Can you work these out from the model? Positions are in its coordinate system, mm. Face numbers are marked on the shaded views. A direction names the side the tool comes from. Give positions to 0.01 mm unless a question says otherwise; leave off trailing zeros. Order: outer loops, then holes, each group sorted by start corner. A loop starts at its lowest first (then second) coordinate and runs counter-clockwise, first axis right, second up. Notation, with made-up numbers: (-16.5, 55) -> (18.5, 55) arc R6 ccw to (18.5, 62) -> close; hole circle Ø8 at (19, 23). An arc over 180 degrees is marked (long way). Answer as CSV lines item,"result".
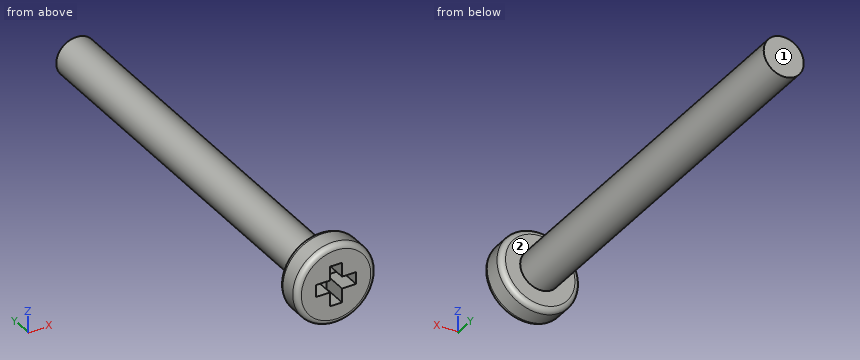
```python
from build123d import *

# Parameters (mm, degrees)
SKETCH1_R           = 3
BOSS_EXTRUDE1_DEPTH = 2
SKETCH2_R           = 1.5
BOSS_EXTRUDE2_DEPTH = 30
SKETCH3_W           = 0.9
SKETCH3_H           = 0.9
SKETCH3_W_2         = 1.05
SKETCH3_H_2         = 1.05
CUT_EXTRUDE1_DEPTH  = 1.9
FILLET1_R           = 0.4


with BuildPart() as part:
    # Sketch1 → Boss-Extrude1 (new body)
    with BuildSketch(Plane(origin=(0, 0, 0), x_dir=(1, 0, 0), z_dir=(0, 1, 0))):
        Circle(SKETCH1_R)
    extrude(amount=BOSS_EXTRUDE1_DEPTH)

    # Sketch2 → Boss-Extrude2 (add)
    with BuildSketch(Plane(origin=(0, 2, 0), x_dir=(1, 0, 0), z_dir=(0, 1, 0))):
        Circle(SKETCH2_R)
    extrude(amount=BOSS_EXTRUDE2_DEPTH)

    # Sketch3 → Cut-Extrude1 (cut)
    with BuildSketch(Plane(origin=(0, 0, 0), x_dir=(-1, 0, 0), z_dir=(0, -1, 0))):
        Rectangle(SKETCH3_W, SKETCH3_H)
        with Locations((0.975, 0)):
            Rectangle(SKETCH3_W_2, SKETCH3_H)
        with Locations((0, -0.975)):
            Rectangle(SKETCH3_W, SKETCH3_H_2)
        with Locations((-0.975, 0)):
            Rectangle(SKETCH3_W_2, SKETCH3_H)
        with Locations((0, 0.975)):
            Rectangle(SKETCH3_W, SKETCH3_H_2)
    extrude(amount=-CUT_EXTRUDE1_DEPTH, mode=Mode.SUBTRACT)

    # Fillet1
    fillet1_edges = [part.edges().sort_by_distance(p)[0] for p in [
        (-3, 0, 0),
        (-3, 2, 0),
    ]]
    fillet(fillet1_edges, radius=FILLET1_R)


solid = part.part
```
Item 1: Imagine slicing it at A-A, the plane z = 0. Please give me the cut outline in (x, y), then the cut area to 3 significant figures.
Numbers:
outline,"(-3, 0.4) arc R0.4 ccw to (-2.6, 0) -> (-1.5, 0) -> (-1.5, 1.9) -> (1.5, 1.9) -> (1.5, 0) -> (2.6, 0) arc R0.4 ccw to (3, 0.4) -> (3, 1.6) arc R0.4 ccw to (2.6, 2) -> (1.5, 2) -> (1.5, 32) -> (-1.5, 32) -> (-1.5, 2) -> (-2.6, 2) arc R0.4 ccw to (-3, 1.6) -> close"
area,"96.2 mm²"
Item 2: Imagine slicing it at C-C, the plane y = 26. Please give me the cut outline in (x, z), then the cut area to 3 significant figures.
Numbers:
outline,"circle Ø3 at (0, 0)"
area,"7.07 mm²"
Item 3: For the marked faces 1 and 2, which set-ups out of +Z, -Z, +X, -X, +Y, -Y let a thin tool reach every point of the face, with its end or its side?
Numbers:
face 1,"+Z, -Z, +X, -X, +Y"
face 2,"+Y"
Item 4: Imagine slicing it at B-B, the plane x = 0. Please give me the cut outline in (y, z).
Numbers:
outline,"(0, -2.6) arc R0.4 ccw to (0.4, -3) -> (1.6, -3) arc R0.4 ccw to (2, -2.6) -> (2, -1.5) -> (32, -1.5) -> (32, 1.5) -> (2, 1.5) -> (2, 2.6) arc R0.4 ccw to (1.6, 3) -> (0.4, 3) arc R0.4 ccw to (0, 2.6) -> (0, 1.5) -> (1.9, 1.5) -> (1.9, -1.5) -> (0, -1.5) -> close"
Item 5: Please list where these lines run through material, in increasing order: line 1 along Y through (x, z) = (1.15, -2.2); line 2 along Y through (x, z) = (0.35, 0.95); line 3 along Z through (x, y) = (0, 25.5).
Numbers:
line 1,"y = 0 to 2"
line 2,"y = 1.9 to 32"
line 3,"z = -1.5 to 1.5"
Item 6: For pin 1 (0.5 mm diameter, centred on x = -1, y = 1, fed in from +Z); pin 2 (0.8 mm diameter, centred on y = 0.5, z = -1, fed in from +X); pin 3 (1.5 mm diameter, centred on x = -1.5, y = 12.5, fed in from -Z); pin 4 (3.5 mm diameter, centred on x = 0, z = 0, fed in from -Y), each with a flat end and sliding along its axis, tell me the tip position at first contact or that it passes through.
Numbers:
pin 1,"stops at z = 2.9"
pin 2,"stops at x = 2.94"
pin 3,"stops at z = -1.3"
pin 4,"stops at y = 0"
